from build123d import *

# Parameters (mm, degrees)
SKETCH1_W           = 330
SKETCH1_H           = 250
BOSS_EXTRUDE1_DEPTH = 6.9
SKETCH2_R           = 3
CUT_EXTRUDE1_DEPTH  = 7.9
SKETCH3_W           = 280
SKETCH3_H           = 200
CUT_EXTRUDE2_DEPTH  = 7.9
FILLET1_R           = 20
FILLET2_R           = 20
CUT_EXTRUDE4_DEPTH  = 7.9


with BuildPart() as part:
    # Sketch1 → Boss-Extrude1 (new body)
    with BuildSketch(Plane(origin=(0, 0, 0), x_dir=(1, 0, 0), z_dir=(0, 1, 0))):
        Rectangle(SKETCH1_W, SKETCH1_H)
    extrude(amount=BOSS_EXTRUDE1_DEPTH)

    # Sketch2 → Cut-Extrude1 (cut, through all)
    with BuildSketch(Plane(origin=(0, 6.9, 0), x_dir=(1, 0, 0), z_dir=(0, 1, 0))):
        with Locations((-145, 105)):
            Circle(SKETCH2_R)
        with Locations((145, 105)):
            Circle(SKETCH2_R)
        with Locations((145, -105)):
            Circle(SKETCH2_R)
        with Locations((-145, -105)):
            Circle(SKETCH2_R)
    extrude(amount=-CUT_EXTRUDE1_DEPTH, mode=Mode.SUBTRACT)

    # Sketch3 → Cut-Extrude2 (cut, through all)
    with BuildSketch(Plane(origin=(0, 6.9, 0), x_dir=(1, 0, 0), z_dir=(0, 1, 0))):
        Rectangle(SKETCH3_W, SKETCH3_H)
    extrude(amount=-CUT_EXTRUDE2_DEPTH, mode=Mode.SUBTRACT)

    # Fillet1
    fillet1_edges = [part.edges().sort_by_distance(p)[0] for p in [
        (-165, 3.45, -125),
        (165, 3.45, -125),
        (165, 3.45, 125),
        (-165, 3.45, 125),
    ]]
    fillet(fillet1_edges, radius=FILLET1_R)

    # Fillet2
    fillet2_edges = [part.edges().sort_by_distance(p)[0] for p in [
        (-140, 3.45, 100),
        (-140, 3.45, -100),
        (140, 3.45, -100),
        (140, 3.45, 100),
    ]]
    fillet(fillet2_edges, radius=FILLET2_R)

    # Sketch4 → Cut-Extrude4 (cut, through all)
    with BuildSketch(Plane(origin=(0, 6.9, 0), x_dir=(1, 0, 0), z_dir=(0, 1, 0))):
        Polygon((-105.386751346, -107.5), (-99.613248654, -107.5), (-96.726497308, -112.5), (-99.613248654, -117.5), (-105.386751346, -117.5), (-108.273502692, -112.5), align=None)
        Polygon((-147.5, -59.613248654), (-152.5, -56.726497308), (-157.5, -59.613248654), (-157.5, -65.386751346), (-152.5, -68.273502692), (-147.5, -65.386751346), align=None)
        Polygon((99.613248654, -107.5), (96.726497308, -112.5), (99.613248654, -117.5), (105.386751346, -117.5), (108.273502692, -112.5), (105.386751346, -107.5), align=None)
        Polygon((147.5, -65.386751346), (147.5, -59.613248654), (152.5, -56.726497308), (157.5, -59.613248654), (157.5, -65.386751346), (152.5, -68.273502692), align=None)
        Polygon((147.5, 59.613248654), (152.5, 56.726497308), (157.5, 59.613248654), (157.5, 65.386751346), (152.5, 68.273502692), (147.5, 65.386751346), align=None)
        Polygon((105.386751346, 107.5), (99.613248654, 107.5), (96.726497308, 112.5), (99.613248654, 117.5), (105.386751346, 117.5), (108.273502692, 112.5), align=None)
        Polygon((-99.613248654, 107.5), (-96.726497308, 112.5), (-99.613248654, 117.5), (-105.386751346, 117.5), (-108.273502692, 112.5), (-105.386751346, 107.5), align=None)
        Polygon((-147.5, 65.386751346), (-147.5, 59.613248654), (-152.5, 56.726497308), (-157.5, 59.613248654), (-157.5, 65.386751346), (-152.5, 68.273502692), align=None)
    extrude(amount=-CUT_EXTRUDE4_DEPTH, mode=Mode.SUBTRACT)


solid = part.part
CAD build for the part. Positions are in the model's coordinates, mm. A direction names the side the tool comes from. Give positions to 0.01 mm unless a question says otherwise; leave off trailing zeros. Write each loop counter-clockwise with the first axis right and the second up, starting at its lowest first coordinate (ties: lowest second). Pieces come first, ordered by that corner, then holes. Notation, with made-up numbers: M 9,29.25 L 26,29.25 A3 cw 26,33.25 Z; hole C 61,35.25 d11. An arc over 180 degrees is marked long. Put each result on its own line as item: value. Start each with the question number.
(1) Probe L1, parallel to X at y = 2.5, z = 105; L2, parallel to Z at x = -145, y = 2.75; L3, parallel to X at y = 6.25, z = -13. List the from-to ranges inside material, lowest first.
(2) Mould opens along X. For faces 1 (the face through (158.986, 3.498, 119.297)), 2 (the face through (-159.297, 3.498, -118.986)), 3 (the face through (-133.986, 3.402, -94.297)), 4 (the face through (140, 3, 1)) say: +X half, -X half, draft (parallel to the pull), parting line (faces both ways), or undercut.
(3) Band-saw the part on C-C, the plane y = 5.5. Give the number of separate pieces and of enclosed holes in the cut face, and give its area (3 significant figures).
(4) Flat gauge pin, fed straight in: pin 1 Ø5 at (x, z) = (-145, -105) entering from +Y. Where does the tip first touch, or does it go through?
(5) Which spindle directions (+Z, -Z, +X, -X, +Y, -Y) get a long thin tool onto all of the face, cutting with end or side? Do faces 5 (the face through (-133.986, 3.402, 94.297)), 6 (the face through (-2, 6.9, 109)). Say none if no direction does.
(6) Band-saw the part on A-A, the plane x = 56. Write the cut outline in (y, z), and give its area (3 significant figures).
(7) Band-saw the part on B-B, the plane z = -4. Write the cut outline in (x, y), and give its area (3 significant figures).
Response values:
1. L1: x = -165 to -148, -142 to 142, 148 to 165
1. L2: z = -125 to -108, -102 to 102, 108 to 125
1. L3: x = -165 to -140, 140 to 165
2. face 1: +X half
2. face 2: -X half
2. face 3: undercut
2. face 4: undercut
3. separate pieces: 1
3. enclosed holes: 13
3. area: 25,700 mm2
4. pin 1: passes through
5. face 5: +Y, -Y
5. face 6: +Z, -Z, +X, -X, +Y
6. outline: M 0,-125 L 6.9,-125 L 6.9,-100 L 0,-100 Z; M 0,100 L 6.9,100 L 6.9,125 L 0,125 Z
6. area: 345 mm2
7. outline: M -165,0 L -140,0 L -140,6.9 L -165,6.9 Z; M 140,0 L 165,0 L 165,6.9 L 140,6.9 Z
7. area: 345 mm2
